Check sheet for the drawn part. Datum: minimum x, y, z corner. Units: mm. Round coordinates to 2 decimals unless told otherwise and drop trailing zeros. Write each loop counter-clockwise with the first axis right and the second up, starting at its lowest first coordinate (ties: lowest second). Pieces come first, ordered by that corner, then holes.
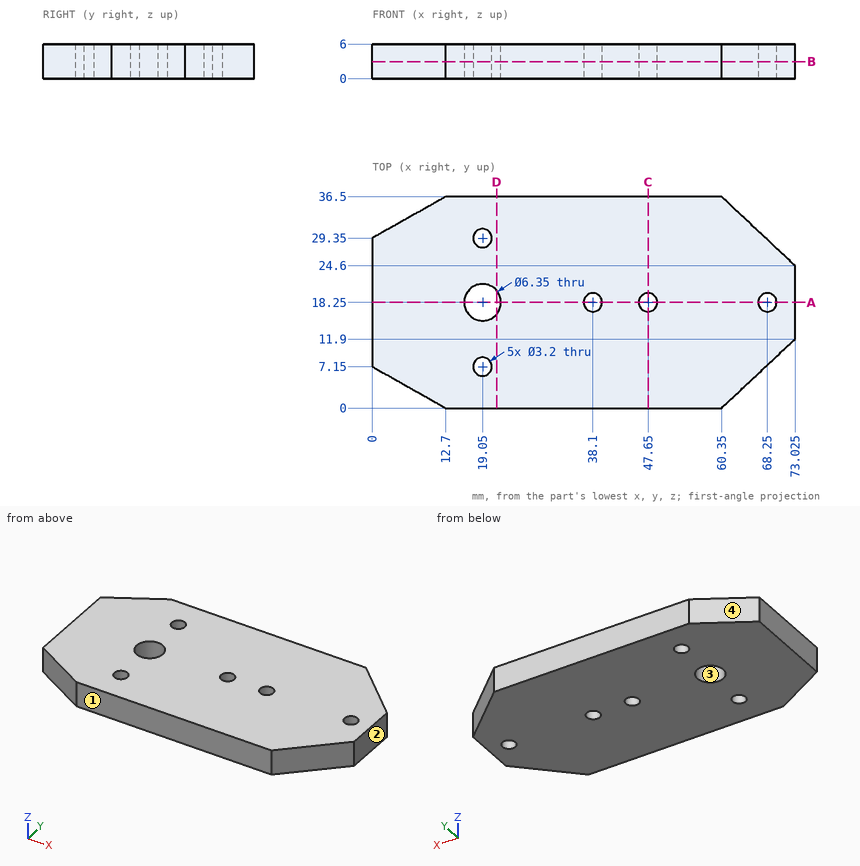
Q1. Sectioned sample at A-A (y = 18.25). Enter the section's corners in (x, z) (3 decimals).
Recorded:
outline: (0, 0) - (15.875, 0) - (15.875, 6) - (0, 6) - close; (22.225, 0) - (36.5, 0) - (36.5, 6) - (22.225, 6) - close; (39.7, 0) - (46.05, 0) - (46.05, 6) - (39.7, 6) - close; (49.25, 0) - (66.65, 0) - (66.65, 6) - (49.25, 6) - close; (69.85, 0) - (73.025, 0) - (73.025, 6) - (69.85, 6) - close
Q2. Material ranges on line 1 along Y through (x, z) = (19.05, 2.9) (3 decimals); line 2 along X through (y, z) = (17, 4.55) (3 decimals); line 3 along Y through (x, z) = (47.65, 2.4), recorded low to high.
Recorded:
line 1: y = 0 to 5.55, 8.75 to 15.075, 21.425 to 27.75, 30.95 to 36.5
line 2: x = 0 to 16.131, 21.969 to 37.101, 39.099 to 46.651, 48.649 to 67.251, 69.249 to 73.025
line 3: y = 0 to 16.65, 19.85 to 36.5
Q3. Sectioned sample at B-B (z = 2.95). Enter the section's corners in (x, y) (3 decimals), plus the area to 3 significant figures.
Recorded:
outline: (0, 7.15) - (12.7, 0) - (60.35, 0) - (73.025, 11.9) - (73.025, 24.6) - (60.35, 36.5) - (12.7, 36.5) - (0, 29.35) - close; hole circle Ø6.35 at (19.05, 18.25); hole circle Ø3.2 at (19.05, 7.15); hole circle Ø3.2 at (19.05, 29.35); hole circle Ø3.2 at (38.1, 18.25); hole circle Ø3.2 at (47.65, 18.25); hole circle Ø3.2 at (68.25, 18.25)
area: 2,350 mm2
Q4. Sectioned sample at C-C (x = 47.65). Enter the section's corners in (y, z).
Recorded:
outline: (0, 0) - (16.65, 0) - (16.65, 6) - (0, 6) - close; (19.85, 0) - (36.5, 0) - (36.5, 6) - (19.85, 6) - close
Q5. Depth check by flat-ended pin: P1, Ø4, axis at x = 50.5, y = 28, coming from the -Z side. Enter the tip coordinate at first touch or a pass-through.
Recorded:
P1: stops at z = 0
Q6. Sectioned sample at D-D (x = 21.5). Enter the section's corners in (y, z), plus the area to 3 significant figures.
Recorded:
outline: (0, 0) - (16.23, 0) - (16.23, 6) - (0, 6) - close; (20.27, 0) - (36.5, 0) - (36.5, 6) - (20.27, 6) - close
area: 195 mm2
Q7. Release check for a two-part mould opening along X. For the marked faces 1, 2, 3 and 4 record: released by +X, released by -X, zero draft, split by the parting line, or undercut.
Recorded:
face 1: zero draft
face 2: released by +X
face 3: undercut
face 4: released by -X
